```python
from build123d import *

# Parameters (mm, degrees)
F0_W     = 227
F0_H     = 75
F1_DEPTH = 7.6


with BuildPart() as f1:
    # F0 (on Top) → F1 (new body)
    with BuildSketch(Plane.XY):
        with BuildLine():
            Line((227, 83), (0, 83))
            ThreePointArc((0, 83), (-5.656854, 80.656854), (-8, 75))
            Line((-8, 75), (-8, 0))
            Line((-8, 0), (-8, -8))
            Line((-8, -8), (0, -8))
            Line((0, -8), (227, -8))
            Line((227, -8), (235, -8))
            Line((235, -8), (235, 0))
            Line((235, 0), (235, 75))
            ThreePointArc((235, 75), (232.656854, 80.656854), (227, 83))
        make_face()
        with Locations((113.5, 37.5)):
            Rectangle(F0_W, F0_H, mode=Mode.SUBTRACT)
    extrude(amount=F1_DEPTH)


solid = f1.part
```
Build history of the part. All positions in model axes, mm. A direction names the side the tool comes from. Round coordinates to 2 decimals unless told otherwise and drop trailing zeros. Loops run counter-clockwise (first coordinate to the right, second up) from the corner with the lowest first, then second, coordinate; pieces in that order, holes last.
Item 1: Saw through at A-A (y = 3). List the corners of the cut face in (x, z), then the cut area to 3 significant figures.
Item 2: Which spindle directions (+Z, -Z, +X, -X, +Y, -Y) get a long thin tool onto all of the face, cutting with end or side? Do faces 4 (the face through (104, -3, 7.6)), 5 (the face through (112, 0, 4)). Say none if no direction does.
Item 3: Drill centre lines: line 1 along X through (y, z) = (11.5, 7); line 2 along Y through (x, z) = (222, 5.5); line 3 along X through (y, z) = (76, 1.25). Where is each one in solid material? Low to high.
Item 4: Two-plate mould, pull along Y, no slides. Class faces 1 (the face through (-8, 34, 4)), 2 (the face through (232.719, 80.594, 3.747)), 3 (the face through (112, 75, 4)): released by +Y, released by -Y, zero draft, split by the parting line, or undercut.
Item 5: Saw through at C-C (z = 5). List the corners of the cut face in (x, y), then the cut area to 3 significant figures.
Item 6: Saw through at B-B (x = 203.5). List the corners of the cut face in (y, z).
Worked answers:
1. outline: (-8, 0) - (0, 0) - (0, 7.6) - (-8, 7.6) - close; (227, 0) - (235, 0) - (235, 7.6) - (227, 7.6) - close
1. area: 122 mm2
2. face 4: +Z, +X, -X, +Y, -Y
2. face 5: +Z, -Z
3. line 1: x = -8 to 0, 227 to 235
3. line 2: y = -8 to 0, 75 to 83
3. line 3: x = -7.94 to 234.94
4. face 1: zero draft
4. face 2: released by +Y
4. face 3: undercut
5. outline: (-8, -8) - (235, -8) - (235, 75) arc R8 ccw to (227, 83) - (0, 83) arc R8 ccw to (-8, 75) - close; hole (0, 0) - (227, 0) - (227, 75) - (0, 75) - close
5. area: 5,060 mm2
6. outline: (-8, 0) - (0, 0) - (0, 7.6) - (-8, 7.6) - close; (75, 0) - (83, 0) - (83, 7.6) - (75, 7.6) - close
